Solid Edge part; units mm, degrees
sketch "Sketch1" plane through (0, 0, 0) normal (0, 0, 1) x (1, 0, 0)
  circle A0 centre (0, 0) radius 5
extrude "Protrusion1" add sketch "Sketch1" along normal blind 2.8
sketch "Sketch2" plane through (0, 0, 0) normal (0, 0, -1) x (1, 0, 0)
  circle A0 centre (0, 0) radius 2.5
extrude "Protrusion2" add sketch "Sketch2" along normal blind 47.2
sketch "Sketch3" plane through (0, 0, -47.2) normal (0, 0, -1) x (1, 0, 0)
  circle A0 centre (0, 0) radius 2.4997
extrude "Cutout1" cut sketch "Sketch3" against normal blind 16 flip side to cut
chamfer "Chamfer_1" distance 0.375 angle 45 1 edges at (-2.4997, 0, -47.2)
sketch "Sketch4" plane through (0, 0, 2.8) normal (0, 0, 1) x (1, 0, 0)
  line L0 (-0.866, 1.5) -> (0.866, 1.5)
  line L1 (1.7321, 0) -> (0.866, 1.5)
  line L2 (0.866, -1.5) -> (1.7321, 0)
  line L3 (-0.866, -1.5) -> (0.866, -1.5)
  line L4 (-1.7321, 0) -> (-0.866, -1.5)
  line L5 (-0.866, 1.5) -> (-1.7321, 0)
extrude "Cutout2" cut sketch "Sketch4" against normal blind 1.8667
sketch "Sketch5" plane through (0, 0, 0) normal (0, -1, 0) x (1, 0, 0)
  line L0 (5, 2.8) -> (2.2, 0)
  line L1 (2.2, 0) -> (5, 0)
  line L2 (5, 0) -> (5, 2.8)
revolve "RevolvedCutout1" cut sketch "Sketch5" angle 360 about axis through (0, 0, 14.0017) along (0, 0, -1)
properties part number "24100000"
For this review, take the finished solid that the model builds, in its own axes (mm). A direction names the side the tool comes from. Give positions to 0.01 mm unless a question says otherwise; leave off trailing zeros. Order: outer loops, then holes, each group sorted by start corner. A loop starts at its lowest first (then second) coordinate and runs counter-clockwise, first axis right, second up. Notation, with made-up numbers: M -14,-23 L 18,-23 A24 cw 18,-2 Z; hole C -38.75,33 d4. An arc over 180 degrees is marked long. Answer in a Markdown table with one row per item. Add a question column.
(1) For pin 1 (3.5 mm diameter, centred on x = -0.5, y = -0.5, fed in from +Z); pin 2 (5 mm diameter, centred on y = -1, z = -8.5, fed in from -X); pin 3 (6 mm diameter, centred on x = 2, z = -11, fed in from -Y); pin 4 (6 mm diameter, centred on y = -3.5, z = -5, fed in from +X), all flat-tipped, find the tip position at first contact; note any pin that passes through.
(2) For faces 1 (the face through (-2, 1.5, -39.1)), 2 (the face through (0, 0, -47.2)), 3 (the face through (1.293, -0.76, 1.88)), list the 3-axis set-ups (+Z, -Z, +X, -X, +Y, -Y) from which the entire face can be reached by the end or side of a thin tool; tool diameter is ignored.
(3) Wall thickness on probe 1 along Y at (x, z) = (2, -25.5); probe 2 along X at (y, z) = (0, -21): over which ranges is each line inside the solid? List them lowest first. Write a range as [from, to].
(4) Consider section B-B on z = -40. State the section outline as (x, y) points, and give its area (3 significant figures).
(5) Mouldability with a two-part tool opening along X and no side actions: class faces 4 (the face through (-0.54, -2.44, -15.38)), 5 (the face through (-1.305, -0.74, 1.88)), 6 (the face through (0, -2, 2.8)) as +X half, -X half, draft (parallel to the pull), parting line (faces both ways), or undercut.
Evaluation:
| question | item | result |
|---|---|---|
| 1 | pin 1 | stops at z = 2.8 |
| 1 | pin 2 | stops at x = -2.5 |
| 1 | pin 3 | stops at y = -2.5 |
| 1 | pin 4 | stops at x = 2.45 |
| 2 | face 1 | -Z |
| 2 | face 2 | -Z, +X, -X, +Y, -Y |
| 2 | face 3 | +Z |
| 3 | probe 1 | y = [-1.5, 1.5] |
| 3 | probe 2 | x = [-2.5, 2.5] |
| 4 | outline | C 0,0 d5 |
| 4 | area | 19.6 mm^2 |
| 5 | face 4 | parting line |
| 5 | face 5 | undercut |
| 5 | face 6 | draft |
